Check sheet for the modelled part. Datum: model origin and axes. Units: mm. A direction names the side the tool comes from. Round coordinates to 2 decimals unless told otherwise and drop trailing zeros. Write each loop counter-clockwise with the first axis right and the second up, starting at its lowest first coordinate (ties: lowest second). Pieces come first, ordered by that corner, then holes. Notation, with made-up numbers: (-1, 62.25) - (31, 62.25) arc R15 cw to (31, 78.25) - close; hole circle Ø4 at (70.25, 1). An arc over 180 degrees is marked (long way). Answer as a JSON object with one key per item and string values. Group by question number.
Item 1: Sectioned sample at D-D on z = 10. Record the boundary of the cut face in (x, y), plus the area to 3 significant figures.
Item 2: Gauge pin test, flat ends, axial feed: P1, Ø15, axis at x = -13, z = -17.5, coming from the +Y side; P2, Ø1.5, axis at x = -4, z = 17, coming from the -Y side; P3, Ø17, axis at x = 1, y = -8.5, coming from the +Z side. Record the tip position at first contact, or that the pin passes through.
Item 3: Thickness scan on line 1 (X direction, y = -7.5, z = 20.5); line 2 (Z direction, x = 19, y = 11); line 3 (Z direction, x = 11, y = 0). Record the ranges inside material, lowest first.
Item 4: Release check for a two-part mould opening along X. For faces 4 (the cylindrical face through (17.871, 17.482, 10.846)), 5 (the cylindrical face through (18.9, -12.7, 9)), 6 (the flat face through (-8.046, -2.967, -4.762)), 7 (the flat face through (-1.8, 4.4, -1.5)) record: pulls with the +X half, pulls with the -X half, needs draft (parallel to the pull), parting line crosses it, or undercut.
Item 5: Set-up check for faces 1 (the flat face through (-4.5, -9, -10.2)), 2 (the flat face through (17, 2, -7)), 3 (the cylindrical face through (-9.9, 18.9, 9)): record each of +Z, -Z, +X, -X, +Y, -Y from which the full face is reachable in a straight line by a thin tool's end or side.
Item 6: Sectioned sample at A-A on z = 2.5. Record the boundary of the cut face in (x, y).
Item 7: Sectioned sample at B-B on y = -17. Record the boundary of the cut face in (x, z).
Item 8: Sectioned sample at C-C on y = -10. Record the boundary of the cut face in (x, z).
```python
from build123d import *

# Parameters (mm, degrees)
BOSS_EXTRUDE1_DEPTH      = 7
EXTRUDE_THIN2_DEPTH      = 15
FILLET1_R                = 7
SKETCH5_W                = 15
SKETCH5_H                = 25
BOSS_EXTRUDE2_DEPTH      = 8
CUT_EXTRUDE2_DEPTH       = 42.641325627
LPATTERN1_COUNT          = 2
LPATTERN1_PITCH          = 26
CHAMFER3_SIZE            = 7
SKETCH9_W                = 15
SKETCH9_H                = 7
BOSS_EXTRUDE3_DEPTH      = 15
BOSS_EXTRUDE4_DEPTH      = 2
BOSS_EXTRUDE4_DEPTH_BACK = 9.9
SKETCH13_W               = 8
SKETCH13_H               = 2
BOSS_EXTRUDE6_DEPTH      = 6
CHAMFER6_SIZE            = 23.744712882
CHAMFER6_SIZE_2          = 13.5
CHAMFER7_SIZE            = 3
SKETCH14_R               = 1.5
CUT_EXTRUDE3_DEPTH       = 15
SKETCH15_W               = 15
SKETCH15_H               = 8.5
CUT_EXTRUDE4_DEPTH       = 6


with BuildPart() as part:
    # Sketch1 → Boss-Extrude1 (new body)
    with BuildSketch(Plane.XY):
        with BuildLine():
            Line((0, 25), (-20, 25))
            Line((-20, 25), (-20, -25))
            Line((-20, -25), (25, -25))
            Line((25, -25), (25, 0))
            ThreePointArc((25, 0), (17.67766953, 17.67766953), (0, 25))
        make_face()
    extrude(amount=BOSS_EXTRUDE1_DEPTH)

    # Sketch3 → Extrude-Thin2 (add)
    with BuildSketch(Plane.XY.offset(7)):
        with BuildLine():
            Line((25, -25), (25, 0))
            ThreePointArc((25, 0), (17.67766953, 17.67766953), (0, 25))
            Line((0, 25), (-20, 25))
            Line((-20, 25), (-20, 21))
            Line((-20, 21), (0, 21))
            ThreePointArc((0, 21), (14.849242405, 14.849242405), (21, 0))
            Line((21, 0), (21, -25))
            Line((21, -25), (25, -25))
        make_face()
    extrude(amount=EXTRUDE_THIN2_DEPTH)

    # Fillet1
    fillet1_edges = [part.edges().sort_by_distance(p)[0] for p in [
        (21, -12.5, 7),
        (14.849242405, 14.849242405, 7),
        (-10, 21, 7),
    ]]
    fillet(fillet1_edges, radius=FILLET1_R)

    # Sketch5 → Boss-Extrude2 (add)
    with BuildSketch(Plane(origin=(25, 0, 0), x_dir=(0, 0, -1), z_dir=(1, 0, 0))):
        with Locations((7.5, -12.5)):
            Rectangle(SKETCH5_W, SKETCH5_H)
    extrude(amount=-BOSS_EXTRUDE2_DEPTH)

    # Sketch8 → Cut-Extrude2 (cut, through all)
    with BuildSketch(Plane.XY.offset(7)):
        with BuildLine():
            Line((-14, -15), (-2, -15))
            ThreePointArc((-2, -15), (0, -17), (-2, -19))
            Line((-2, -19), (-14, -19))
            ThreePointArc((-14, -19), (-16, -17), (-14, -15))
        make_face()
    cut_extrude2 = extrude(amount=-CUT_EXTRUDE2_DEPTH, mode=Mode.SUBTRACT)

    # LPattern1: Cut-Extrude2 ×2
    with Locations(*[(0, i * LPATTERN1_PITCH, 0) for i in range(1, LPATTERN1_COUNT)]):
        add(cut_extrude2, mode=Mode.SUBTRACT)

    # Chamfer3
    chamfer3_edges = [part.edges().sort_by_distance(p)[0] for p in [
        (25, -12.5, -15),
    ]]
    chamfer(chamfer3_edges, length=CHAMFER3_SIZE)

    # Sketch9 → Boss-Extrude3 (add)
    with BuildSketch(Plane.ZY.offset(-17)):
        with Locations((-7.5, -3.5)):
            Rectangle(SKETCH9_W, SKETCH9_H)
    extrude(amount=BOSS_EXTRUDE3_DEPTH)

    # Sketch10 → Boss-Extrude4 (add, two sides: drawn at the far end of the back side and taken through both)
    with BuildSketch(Plane.XZ.offset(7).offset(-BOSS_EXTRUDE4_DEPTH_BACK)):
        Polygon((2, -15), (-6.970562748, -15), (-12.627416998, -9.343145751), (-16.870057685, -13.585786438), (-20, -10.455844123), (-20, 0), (17, 0), (17, -15), align=None)
        Polygon((-4.849242405, -10.050252532), (-9.091883092, -5.807611845), (-6.970562748, -3.686291501), (-2.727922061, -7.928932188), align=None, mode=Mode.SUBTRACT)
    extrude(amount=BOSS_EXTRUDE4_DEPTH + BOSS_EXTRUDE4_DEPTH_BACK)

    # Sketch13 → Boss-Extrude6 (add)
    with BuildSketch(Plane(origin=(-10.985281374, 0, -10.985281374), x_dir=(-0.7071067811865478, 0, 0.7071067811865472), z_dir=(-0.7071067811865472, 0, -0.7071067811865478))):
        with Locations((-1.67766953, 1.9)):
            Rectangle(SKETCH13_W, SKETCH13_H)
        with Locations((-1.67766953, -8)):
            Rectangle(SKETCH13_W, SKETCH13_H)
    extrude(amount=BOSS_EXTRUDE6_DEPTH)

    # Chamfer6
    # the kernel refuses this chamfer: 23.744712882, 13.5 mm, written as the material it adds along each edge
    with BuildSketch(Plane(origin=(-6.970562748, -9, -15), x_dir=(-0.7145740403020574, 0, -0.6995598194053126), z_dir=(0, 1, 0))) as chamfer6_piece_1_section:
        Polygon((CHAMFER6_SIZE * 0.999943641689, -CHAMFER6_SIZE * 0.0106166574102), (-CHAMFER6_SIZE_2 * 0.714574040302, -CHAMFER6_SIZE_2 * 0.699559819405), (0, 0), align=None)
    chamfer6_piece_1 = extrude(amount=2, mode=Mode.PRIVATE)
    chamfer6_piece_1 = split(chamfer6_piece_1, bisect_by=Plane(origin=(-9.095447466, -8, -21.360396657), z_dir=(0.7071067811865476, 0, 0.7071067811865476)), keep=Keep.TOP, mode=Mode.PRIVATE)
    add(chamfer6_piece_1)
    with BuildSketch(Plane(origin=(-6.970562748, -70.647744863, -15), x_dir=(-0.7145740403020574, 0, -0.6995598194053126), z_dir=(0, 1, 0))) as chamfer6_piece_2_section:
        Polygon((CHAMFER6_SIZE * 0.999943641689, -CHAMFER6_SIZE * 0.0106166574102), (-CHAMFER6_SIZE_2 * 0.714574040302, -CHAMFER6_SIZE_2 * 0.699559819405), (0, 0), align=None)
    chamfer6_piece_2 = extrude(amount=125.295489727, mode=Mode.PRIVATE)
    chamfer6_piece_2 = split(chamfer6_piece_2, bisect_by=Plane(origin=(-6.871868761, 2.9, -19.136817952), z_dir=(0, -1, 0)), keep=Keep.TOP, mode=Mode.PRIVATE)
    chamfer6_piece_2 = split(chamfer6_piece_2, bisect_by=Plane(origin=(-6.871868761, 0.9, -19.136817952), z_dir=(0, 1, 0)), keep=Keep.TOP, mode=Mode.PRIVATE)
    chamfer6_piece_2 = split(chamfer6_piece_2, bisect_by=Plane(origin=(-9.095447466, 1.9, -21.360396657), z_dir=(0.7071067811865476, 0, 0.7071067811865476)), keep=Keep.TOP, mode=Mode.PRIVATE)
    add(chamfer6_piece_2)
    with BuildSketch(Plane(origin=(-6.970562748, -60.747744863, -15), x_dir=(-0.7145740403020574, 0, -0.6995598194053126), z_dir=(0, 1, 0))) as chamfer6_piece_3_section:
        Polygon((CHAMFER6_SIZE * 0.999943641689, -CHAMFER6_SIZE * 0.0106166574102), (-CHAMFER6_SIZE_2 * 0.714574040302, -CHAMFER6_SIZE_2 * 0.699559819405), (0, 0), align=None)
    chamfer6_piece_3 = extrude(amount=125.295489727, mode=Mode.PRIVATE)
    chamfer6_piece_3 = split(chamfer6_piece_3, bisect_by=Plane(origin=(-6.871868761, -7, -19.136817952), z_dir=(0, -1, 0)), keep=Keep.TOP, mode=Mode.PRIVATE)
    chamfer6_piece_3 = split(chamfer6_piece_3, bisect_by=Plane(origin=(-9.095447466, -8, -21.360396657), z_dir=(0.7071067811865476, 0, 0.7071067811865476)), keep=Keep.TOP, mode=Mode.PRIVATE)
    chamfer6_piece_3 = split(chamfer6_piece_3, bisect_by=Plane(origin=(-6.871868761, -9, -19.136817952), z_dir=(0, 1, 0)), keep=Keep.TOP, mode=Mode.PRIVATE)
    add(chamfer6_piece_3)
    with BuildSketch(Plane(origin=(-6.970562748, 0.9, -15), x_dir=(-0.7145740403020574, 0, -0.6995598194053126), z_dir=(0, 1, 0))) as chamfer6_piece_4_section:
        Polygon((CHAMFER6_SIZE * 0.999943641689, -CHAMFER6_SIZE * 0.0106166574102), (-CHAMFER6_SIZE_2 * 0.714574040302, -CHAMFER6_SIZE_2 * 0.699559819405), (0, 0), align=None)
    chamfer6_piece_4 = extrude(amount=2, mode=Mode.PRIVATE)
    chamfer6_piece_4 = split(chamfer6_piece_4, bisect_by=Plane(origin=(-9.095447466, 1.9, -21.360396657), z_dir=(0.7071067811865476, 0, 0.7071067811865476)), keep=Keep.TOP, mode=Mode.PRIVATE)
    add(chamfer6_piece_4)

    # Chamfer7
    chamfer7_edges = [part.edges().sort_by_distance(p)[0] for p in [
        (-1.5, 2.9, 0),
        (17, -9, -7.5),
        (17, -17, 0),
        (-1.5, -9, 0),
    ]]
    chamfer(chamfer7_edges, length=CHAMFER7_SIZE)

    # Sketch14 → Cut-Extrude3 (cut)
    with BuildSketch(Plane(origin=(-10.985281374, 0, -10.985281374), x_dir=(-0.7071067811865478, 0, 0.7071067811865472), z_dir=(-0.7071067811865472, 0, -0.7071067811865478))):
        with Locations((-0.67766953, -3.05)):
            Circle(SKETCH14_R)
    extrude(amount=-CUT_EXTRUDE3_DEPTH, mode=Mode.SUBTRACT)

    # Sketch15 → Cut-Extrude4 (cut)
    with BuildSketch(Plane(origin=(-15.227922061, 0, -15.227922061), x_dir=(-0.7071067811865475, 0, 0.7071067811865477), z_dir=(-0.7071067811865477, 0, -0.7071067811865475))):
        with Locations((-4.87766953, -3.05)):
            Rectangle(SKETCH15_W, SKETCH15_H)
    extrude(amount=-CUT_EXTRUDE4_DEPTH, mode=Mode.SUBTRACT)


solid = part.part
```
Completed:
{
 "1": {"outline": "(-20, 19.74) - (0, 19.74) arc R19.74 cw to (19.74, 0) - (19.74, -25) - (25, -25) - (25, 0) arc R25 ccw to (0, 25) - (-20, 25) - close", "area": "421 mm²"},
 "2": {"P1": "y = 2.9", "P2": "y = 21", "P3": "z = 7"},
 "3": {"line 1": "21 to 25", "line 2": "0 to 22", "line 3": "-15 to 7"},
 "4": {"face 4": "pulls with the +X half", "face 5": "pulls with the -X half", "face 6": "undercut", "face 7": "needs draft"},
 "5": {"face 1": "-Z, -X, -Y", "face 2": "-Z, +X, +Y", "face 3": "+Z, -X, -Y"},
 "6": {"outline": "(-20, -25) - (25, -25) - (25, 0) arc R25 ccw to (0, 25) - (-20, 25) - close; hole (-14, -19) - (-2, -19) arc R2 ccw to (-2, -15) - (-14, -15) arc R2 ccw to start; hole (-14, 7) - (-2, 7) arc R2 ccw to (-2, 11) - (-14, 11) arc R2 ccw to start"},
 "7": {"outline": "(-20, 0) - (-16, 0) - (-16, 7) - (-20, 7) - close; (0, 0) - (14, 0) - (17, -3) - (17, -15) - (18, -15) - (25, -8) - (25, 22) - (21, 22) - (21, 14) arc R7 cw to (14, 7) - (0, 7) - close"},
 "8": {"outline": "(-20, -2) - (14, -2) - (15, -3) - (15, -15) - (18, -15) - (25, -8) - (25, 22) - (21, 22) - (21, 14) arc R7 cw to (14, 7) - (-20, 7) - close"}
}
